Here's how the part is built. I have some questions about the finished solid (model axes, mm). Face numbers are marked on the shaded views. A direction names the side the tool comes from. Give positions to 0.01 mm unless a question says otherwise; leave off trailing zeros. Loops run counter-clockwise (first coordinate to the right, second up) from the corner with the lowest first, then second, coordinate; pieces in that order, holes last. Notation, with made-up numbers: (-17.75, 69) - (12.25, 69) arc R26 ccw to (12.25, 102) - close; hole circle Ø1 at (-13, -21). An arc over 180 degrees is marked (long way). One line per item, written item: value. Start each with the question number.
```python
from build123d import *

# Parameters (mm, degrees)
BOSS_EXTRUDE1_DEPTH     = 12
CUT_EXTRUDE1_DEPTH      = 36.397740041
CUT_EXTRUDE1_DEPTH_BACK = 36.397740041
SKETCH2_R               = 3.15
CUT_EXTRUDE2_REACH      = 34.527
SKETCH3_R               = 1.4


with BuildPart() as part:
    # Sketch1 → Boss-Extrude1 (new body)
    with BuildSketch(Plane.XY):
        with BuildLine():
            Line((10, 6), (22, 6))
            Line((22, 6), (22, 2.552710574))
            Line((22, 2.552710574), (2.091331807, 2.552710574))
            ThreePointArc((2.091331807, 2.552710574), (-3.3, 0), (2.091331807, -2.552710574))
            Line((2.091331807, -2.552710574), (22, -2.552710574))
            Line((22, -2.552710574), (22, -6))
            Line((22, -6), (0, -6))
            ThreePointArc((0, -6), (-6, 0), (0, 6))
            Line((0, 6), (5, 6))
            Line((5, 6), (5, 25))
            Line((5, 25), (8, 25))
            Line((8, 25), (8, 8))
            ThreePointArc((8, 8), (8.585786438, 6.585786438), (10, 6))
        make_face()
    extrude(amount=BOSS_EXTRUDE1_DEPTH)

    # Sketch2 → Cut-Extrude1 (cut, two sides: drawn at the far end of the back side and taken through both)
    with BuildSketch(Plane(origin=(0, 0, 0), x_dir=(1, 0, 0), z_dir=(0, 1, 0)).offset(-CUT_EXTRUDE1_DEPTH_BACK)):
        with Locations(Location((16, -6, 0), (0, 0, 270))):
            Circle(SKETCH2_R)
    extrude(amount=CUT_EXTRUDE1_DEPTH + CUT_EXTRUDE1_DEPTH_BACK, mode=Mode.SUBTRACT)

    # Sketch3 → Cut-Extrude2 (cut, up to next)
    with BuildSketch(Plane.ZY.offset(-5), mode=Mode.PRIVATE) as cut_extrude2_sk1:
        with Locations((6, 21)):
            Circle(SKETCH3_R)
    cut_extrude2_tool1 = extrude(cut_extrude2_sk1.sketch, amount=-CUT_EXTRUDE2_REACH, mode=Mode.PRIVATE) & part.part
    # Sketch3 → Cut-Extrude2 (cut, up to next)
    with BuildSketch(Plane.ZY.offset(-5), mode=Mode.PRIVATE) as cut_extrude2_sk2:
        with Locations((6, 11.5)):
            Circle(SKETCH3_R)
    cut_extrude2_tool2 = extrude(cut_extrude2_sk2.sketch, amount=-CUT_EXTRUDE2_REACH, mode=Mode.PRIVATE) & part.part
    add(cut_extrude2_tool1.solids().sort_by_distance((5, 21, 6))[0], mode=Mode.SUBTRACT)
    add(cut_extrude2_tool2.solids().sort_by_distance((5, 11.5, 6))[0], mode=Mode.SUBTRACT)


solid = part.part
```
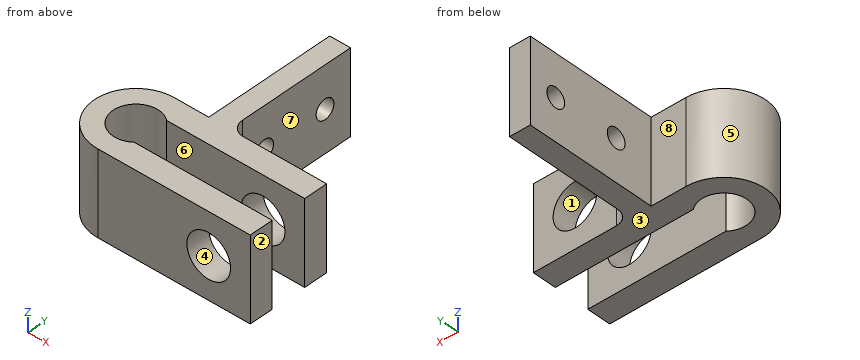
(1) If we section it at C-C on z = 6: Give the number of separate pieces and of enclosed holes in the cut face, plus the area to 3 significant figures.
(2) If we section it at D-D on x = 4.25: List the corners of the cut face in (y, z) for me.
(3) If we section it at B-B on x = 16: List the corners of the cut face in (y, z) for me, plus the area to 3 significant figures.
(4) Please list where these lines run through material, in increasing order: probe 1 along Y at (x, z) = (6.8, 6); probe 2 along Y at (x, z) = (15.25, 9.25); probe 3 along Z at (x, y) = (16, -5). Write a range as from..to.
(5) If we mould it in two halves opening along Z, with no side actions, what happens to the marked faces 1, 2, 3 and 4? For each: pulls with the +Z half, pulls with the -Z half, needs draft (parallel to the pull), parting line crosses it, or undercut.
(6) If we section it at A-A on y = 11.5: List the corners of the cut face in (x, z) for me, plus the area to 3 significant figures.
(7) For the marked faces 5, 6, 7 and 8, which set-ups out of +Z, -Z, +X, -X, +Y, -Y let a thin tool reach every point of the face, with its end or its side?
(8) Will these pins go through, and if not, where does the flat tip stop? pin 1 (5.5 mm diameter, centred on x = 1.5, z = 8, fed in from +Y); pin 2 (6 mm diameter, centred on y = 15.5, z = 6, fed in from +X); pin 3 (6 mm diameter, centred on y = 12, z = 7.5, fed in from -X).
Found:
1. separate pieces: 5
1. enclosed holes: 0
1. area: 187 mm^2
2. outline: (-6, 0) - (-2.55, 0) - (-2.55, 12) - (-6, 12) - close; (2.55, 0) - (6, 0) - (6, 12) - (2.55, 12) - close
3. outline: (-6, 0) - (-2.55, 0) - (-2.55, 2.85) - (-6, 2.85) - close; (-6, 9.15) - (-2.55, 9.15) - (-2.55, 12) - (-6, 12) - close; (2.55, 0) - (6, 0) - (6, 2.85) - (2.55, 2.85) - close; (2.55, 9.15) - (6, 9.15) - (6, 12) - (2.55, 12) - close
3. area: 39.3 mm^2
4. probe 1: -6..-2.55, 2.55..10.1, 12.9..19.6, 22.4..25
4. probe 2: -6..-2.55, 2.55..6
4. probe 3: 0..2.85, 9.15..12
5. face 1: undercut
5. face 2: needs draft
5. face 3: pulls with the -Z half
5. face 4: undercut
6. outline: (5, 0) - (8, 0) - (8, 4.6) - (5, 4.6) - close; (5, 7.4) - (8, 7.4) - (8, 12) - (5, 12) - close
6. area: 27.6 mm^2
7. face 5: +Z, -Z, -X
7. face 6: +Z, -Z, +X
7. face 7: +Z, -Z, +X, +Y
7. face 8: +Z, -Z, -X, +Y
8. pin 1: y = 6
8. pin 2: x = 8
8. pin 3: x = 5
